Part model, mm, in its own coordinate system. A direction names the side the tool comes from. Coordinates: 2 decimals unless noted, no trailing zeros. Loops run counter-clockwise (first coordinate to the right, second up) from the corner with the lowest first, then second, coordinate; pieces in that order, holes last. Notation, with made-up numbers: (11.5, 40.5) -> (50.5, 40.5) arc R30 ccw to (50.5, 78.5) -> close; hole circle Ø5 at (40.25, 44). An arc over 180 degrees is marked (long way). Use one line per item in the form item = value. Start each with the question number.
(1) Band-saw the part on B-B on z = 3.25. Give the cut face in (x, y).
(2) Band-saw the part on A-A on x = 26. Give the cut face in (y, z), then the cut area to 3 significant figures.
(3) Mould opens along Y. For faces 3 (the cylindrical face through (6, 22, 5)), 4 (the flat face through (16, 27, 5)), 5 (the flat face through (16, 4, 9.8)) say: +Y half, -Y half, draft (parallel to the pull), parting line (faces both ways), or undercut.
(4) Drill centre lines: L1, parallel to X at y = 23.5, z = 7.5; L2, parallel to Y at x = 6, z = 3.5; L3, parallel to X at y = 24.25, z = 9.25. Where is each one in solid material? Low to high. Write a range as [from, to].
(5) Band-saw the part on C-C on y = 3.5. Give the cut face in (x, z), then the cut area to 3 significant figures.
(6) 3-axis set-ups, long thin cutter, end or side, ignore diameter. For faces 1 (the flat face through (16, 0, 5)), 2 (the flat face through (16, 7.5, 7)): which of +Z, -Z, +X, -X, +Y, -Y reach the whole face in a straight line?
(7) Band-saw the part on D-D on x = 21.5. Give the cut face in (y, z).
Autodesk Fusion 360 part; units mm, degrees
sketch "Sketch1" plane through (0, 0, 0) normal (0, 0, 1) x (1, 0, 0)
  line L0 (0, 0) -> (32, 0)
  line L1 (32, 0) -> (32, 27)
  line L2 (32, 27) -> (0, 27)
  line L3 (0, 27) -> (0, 0)
  dimension "d1" = 27
  dimension "d2" = 32
extrude "Extrude1" add sketch "Sketch1" along normal blind 4.8
sketch "Sketch2" plane through (0, 0, 4.8) normal (0, 0, 1) x (-1, 0, 0)
  line L0 (0, -27) -> (0, 0)
  line L1 (0, 0) -> (-32, 0)
  line L2 (-32, 0) -> (-32, -27)
  line L3 (-32, -27) -> (0, -27)
  line L4 (0, 0) -> (-32, 0)
  line L5 (-32, 0) -> (-32, -7.5)
  line L6 (-32, -7.5) -> (0, -7.5)
  line L7 (0, -7.5) -> (0, 0)
  line L8 (-32, -27) -> (0, -27)
  line L9 (0, -27) -> (0, -19.5)
  line L10 (0, -19.5) -> (-32, -19.5)
  line L11 (-32, -19.5) -> (-32, -27)
  dimension "d5" = 12
  dimension "d6" = 7.5
  dimension "d7" = 8.2363
extrude "Extrude2" add sketch "Sketch2" along normal blind 5 contours L0 L2 L3 L8 L9 L10 L11 | L0 L1 L2 L4 L5 L6 L7
sketch "Sketch3" plane through (0, 0, 0) normal (0, 0, -1) x (1, 0, 0)
  line L0 (0, 0) -> (0, -27)
  line L1 (0, -27) -> (32, -27)
  line L2 (32, -27) -> (32, 0)
  line L3 (32, 0) -> (0, 0)
  line L4 (6, -3.5) -> (26, -3.5)
  line L5 (26, -3.5) -> (26, -23.5)
  line L6 (26, -23.5) -> (6, -23.5)
  line L7 (6, -23.5) -> (6, -3.5)
  circle A0 centre (6, -3.5) radius 1.5
  circle A1 centre (26, -3.5) radius 1.5
  circle A2 centre (6, -23.5) radius 1.5
  circle A3 centre (26, -23.5) radius 1.5
  dimension "d10" = 20
  dimension "d11" = 20
  dimension "d12" = 3.5
  dimension "d13" = 3
  dimension "d14" = 6
  dimension "d15" = 6
  dimension "d16" = 3
  dimension "d17" = 3
  dimension "d18" = 3
  dimension "d19" = 3
extrude "Extrude3" cut sketch "Sketch3" against normal blind 20 contours L4 L7 A0 | L4 L7 A0 | L4 L5 A1 | L4 L5 A1 | L6 L7 A2 | L6 L7 A2 | L5 L6 A3 | L5 L6 A3
chamfer "Chamfer1" distance 0.25 angle 45 4 edges at (4.6015, 2.9576, 0) (24.6015, 2.9576, 0) (24.6015, 22.9576, 0) (4.6015, 22.9576, 0)
thread "Thread1"
A:
q1.outline = (0, 0) -> (32, 0) -> (32, 27) -> (0, 27) -> close; hole circle Ø3 at (6, 3.5); hole circle Ø3 at (6, 23.5); hole circle Ø3 at (26, 3.5); hole circle Ø3 at (26, 23.5)
q2.outline = (0, 0) -> (1.75, 0) -> (2, 0.25) -> (2, 9.8) -> (0, 9.8) -> close; (5, 0.25) -> (5.25, 0) -> (21.75, 0) -> (22, 0.25) -> (22, 9.8) -> (19.5, 9.8) -> (19.5, 4.8) -> (7.5, 4.8) -> (7.5, 9.8) -> (5, 9.8) -> close; (25, 0.25) -> (25.25, 0) -> (27, 0) -> (27, 9.8) -> (25, 9.8) -> close
q2.area = 146 mm²
q3.face_3 = undercut
q3.face_4 = +Y half
q3.face_5 = draft
q4.L1 = [0, 4.5], [7.5, 24.5], [27.5, 32]
q4.L2 = [0, 2], [5, 22], [25, 27]
q4.L3 = [0, 4.7], [7.3, 24.7], [27.3, 32]
q5.outline = (0, 0) -> (4.25, 0) -> (4.5, 0.25) -> (4.5, 9.8) -> (0, 9.8) -> close; (7.5, 0.25) -> (7.75, 0) -> (24.25, 0) -> (24.5, 0.25) -> (24.5, 9.8) -> (7.5, 9.8) -> close; (27.5, 0.25) -> (27.75, 0) -> (32, 0) -> (32, 9.8) -> (27.5, 9.8) -> close
q5.area = 255 mm²
q6.face_1 = +Z, -Z, +X, -X, -Y
q6.face_2 = +Z, +X, -X
q7.outline = (0, 0) -> (27, 0) -> (27, 9.8) -> (19.5, 9.8) -> (19.5, 4.8) -> (7.5, 4.8) -> (7.5, 9.8) -> (0, 9.8) -> close
